Could you check a few things on this drawing? It's one solid part, dimensions in mm from its lowest x, y, z. Coordinates: 2 decimals unless noted, no trailing zeros. Write each loop counter-clockwise with the first axis right and the second up, starting at its lowest first coordinate (ties: lowest second). Pieces come first, ordered by that corner, then holes.
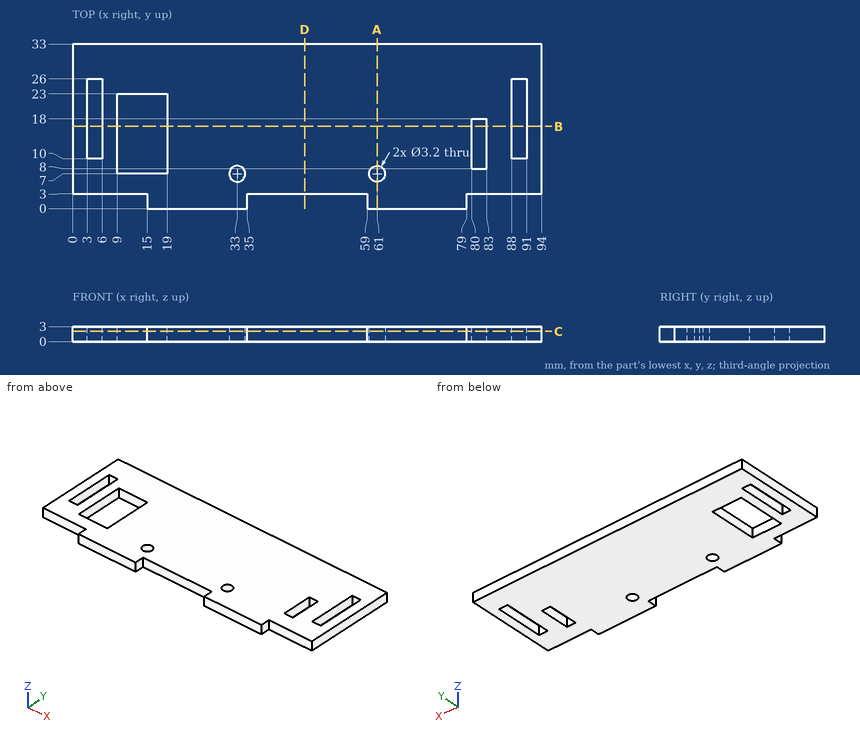
1) Imagine slicing it at D-D on x = 46.5. Please give me the cut outline in (y, z), then the cut area to 3 significant figures.
Values follow:
outline: (3, 0) - (33, 0) - (33, 3) - (3, 3) - close
area: 90.0 mm2
2) Imagine slicing it at B-B on y = 16.5. Please give me the cut outline in (x, z), then the cut area to 3 significant figures.
Values follow:
outline: (0, 0) - (3, 0) - (3, 3) - (0, 3) - close; (6, 0) - (9, 0) - (9, 3) - (6, 3) - close; (19, 0) - (80, 0) - (80, 3) - (19, 3) - close; (83, 0) - (88, 0) - (88, 3) - (83, 3) - close; (91, 0) - (94, 0) - (94, 3) - (91, 3) - close
area: 225 mm2
3) I need wall thicknesses on probe 1 along X at (y, z) = (25, 0.4); probe 2 along X at (y, z) = (15, 2.4); probe 3 along Y at (x, z) = (61, 1.4). Which ranges of each line are inside material? Lowest first, please.
Values follow:
probe 1: x = 0 to 3, 6 to 88, 91 to 94
probe 2: x = 0 to 3, 6 to 9, 19 to 80, 83 to 88, 91 to 94
probe 3: y = 0 to 5.4, 8.6 to 33
4) Imagine slicing it at A-A on x = 61. Please give me the cut outline in (y, z), then the cut area to 3 significant figures.
Values follow:
outline: (0, 0) - (5.4, 0) - (5.4, 3) - (0, 3) - close; (8.6, 0) - (33, 0) - (33, 3) - (8.6, 3) - close
area: 89.4 mm2
5) Imagine slicing it at C-C on z = 2.05. Count the separate pieces of the cut face and the enclosed holes in it, then the cut area to 3 significant figures.
Values follow:
separate pieces: 1
enclosed holes: 6
area: 2,640 mm2
6) Will these pins go through, and if not, where does the flat tip stop? pin 1 (1.5 mm diameter, centred on y = 1, z = 2, fed in from +X); pin 2 (0.9 mm diameter, centred on x = 83.5, z = 1, fed in from -Y).
Values follow:
pin 1: stops at x = 79
pin 2: stops at y = 3
